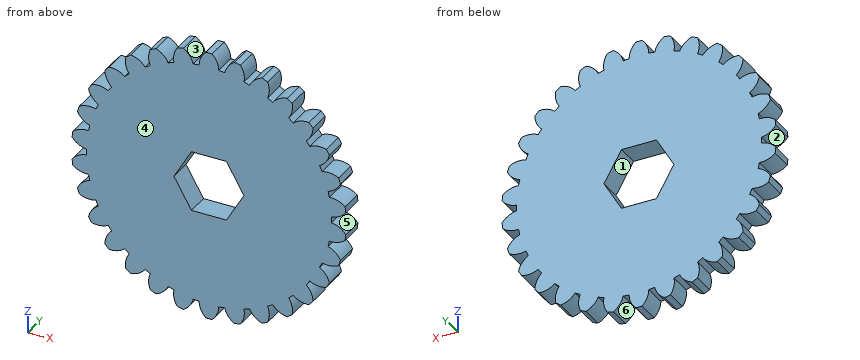
```python
from build123d import *

# Parameters (mm, degrees)
SKETCH2_R           = 25.664173075
BOSS_EXTRUDE2_DEPTH = 4.7625
BOSS_EXTRUDE3_DEPTH = 4.7625
CIRPATTERN1_COUNT   = 30


with BuildPart() as part:
    # Sketch2 → Boss-Extrude2 (new body)
    with BuildSketch(Plane(origin=(0, 0, 0), x_dir=(1, 0, 0), z_dir=(0, 1, 0))):
        Circle(SKETCH2_R)
        Polygon((7.332348419, 0), (3.666174209, 6.35), (-3.666174209, 6.35), (-7.332348419, 0), (-3.666174209, -6.35), (3.666174209, -6.35), align=None, mode=Mode.SUBTRACT)
    extrude(amount=BOSS_EXTRUDE2_DEPTH)

    # Sketch1 → Boss-Extrude3 (add)
    with BuildSketch(Plane(origin=(0, 0, 0), x_dir=(1, 0, 0), z_dir=(0, 1, 0))):
        with BuildLine():
            Line((0.640211275, 28.764979636), (-0.640211275, 28.764979636))
            ThreePointArc((-0.640211275, 28.764979636), (-1.726312193, 27.213866774), (-2.055125292, 25.349075026))
            ThreePointArc((-2.055125292, 25.349075026), (0, 25.432246157), (2.055125292, 25.349075026))
            ThreePointArc((2.055125292, 25.349075026), (1.726312193, 27.213866774), (0.640211275, 28.764979636))
        make_face()
    boss_extrude3 = extrude(amount=BOSS_EXTRUDE3_DEPTH)

    # CirPattern1: Boss-Extrude3 ×30 about axis
    cirpattern1_axis = Axis((0, 0, 0), (0, 1, 0))
    for i in range(1, CIRPATTERN1_COUNT):
        add(boss_extrude3.rotate(cirpattern1_axis, i * 360 / CIRPATTERN1_COUNT))


solid = part.part
```
Here's how the part is built. I have some questions about the finished solid (model axes, mm). Face numbers are marked on the shaded views. A direction names the side the tool comes from. Give positions to 0.01 mm unless a question says otherwise; leave off trailing zeros. Order: outer loops, then holes, each group sorted by start corner. A loop starts at its lowest first (then second) coordinate and runs counter-clockwise, first axis right, second up. Notation, with made-up numbers: M -8,-10.5 L 1,-10.5 A27 ccw 1,20.5 Z; hole C -29,2 d4. An arc over 180 degrees is marked long. Use a Markdown table: item, result. Add a question column.
1. Suppose I cut it at A-A (z = 12). List the corners of the cut face in (x, y) for me.
2. For pin 1 Ø10 at (x, z) = (18, 7) entering from -Y; pin 2 Ø1 at (x, y) = (-1.5, 2.5) entering from -Z, each with a flat end and sliding along its axis, tell me the tip position at first contact or that it passes through.
3. On a 3-axis mill with a long thin cutter (end or side, diameter ignored), from which of +Z, -Z, +X, -X, +Y, -Y can I reach the whole of each face in a straight line? I mean the marked faces 1, 2 and 3. Say none if no direction works.
4. If we mould it in two halves opening along X, with no side actions, what happens to the marked faces 4, 5 and 6? For each: +X half, -X half, draft (parallel to the pull), parting line (faces both ways), or undercut.
5. I need wall thicknesses on probe 1 along X at (y, z) = (4.05, 22); probe 2 along Z at (x, y) = (26, 3.7); probe 3 along Z at (x, y) = (-24, 2.9). Which ranges of each line are inside material? Lowest first, please. Write a range as from..to.
Results list:
| question | item | result |
|---|---|---|
| 1 | outline | M -24.34,0 L 24.34,0 L 24.34,4.76 L -24.34,4.76 Z |
| 2 | pin 1 | stops at y = 0 |
| 2 | pin 2 | stops at z = -28.39 |
| 3 | face 1 | +Y, -Y |
| 3 | face 2 | -X, +Y, -Y |
| 3 | face 3 | +Z, +Y, -Y |
| 4 | face 4 | draft |
| 4 | face 5 | +X half |
| 4 | face 6 | undercut |
| 5 | probe 1 | x = -17.51..-13.44, -13.22..13.22, 13.44..17.51 |
| 5 | probe 2 | z = -9.95..-6.45, -4.73..-0.68, 0.68..4.73, 6.45..9.95 |
| 5 | probe 3 | z = -15.08..-11.63, -9.95..9.95, 11.63..15.08 |
